Input: part model. Units: mm. Frame: model coordinates. Coordinates: 2 decimals unless noted, no trailing zeros. Write each loop counter-clockwise with the first axis right and the second up, starting at its lowest first coordinate (ties: lowest second). Pieces come first, ordered by that corner, then holes. Notation, with made-up numbers: M 52,83 L 107,83 A19 cw 107,95 Z; hole C 30,51 d6. An arc over 180 degrees is marked long. Use one line per item in the form item = value.
from build123d import *

# Parameters (mm, degrees)
SKETCH_1_W             = 270
SKETCH_1_H             = 107
SM_BASE_FLANGE_1_DEPTH = 5
SKETCH_6_R             = 3
CUT_EXTRUDE_1_DEPTH    = 10
SKETCH_7_R             = 1.5
CUT_EXTRUDE_2_DEPTH    = 10
FILLET_1_R             = 1
SKETCH_8_R             = 1.5
CUT_EXTRUDE_3_DEPTH    = 10


# Sheet-metal steps are written as plain solids
with BuildPart() as part:
    # Sketch 1 → 基体-法兰1 (new body)
    with BuildSketch(Plane.XY):
        Rectangle(SKETCH_1_W, SKETCH_1_H)
    extrude(amount=-SM_BASE_FLANGE_1_DEPTH)

    # 草图6 → 切除-拉伸1 (cut)
    with BuildSketch(Plane.XY):
        with Locations((-129, 35.5)):
            Circle(SKETCH_6_R)
        with Locations((-129, -35.5)):
            Circle(SKETCH_6_R)
        with Locations((-85, 35.5)):
            Circle(SKETCH_6_R)
        with Locations((-85, -35.5)):
            Circle(SKETCH_6_R)
    cut_extrude_1 = extrude(amount=-CUT_EXTRUDE_1_DEPTH, mode=Mode.SUBTRACT)

    # 镜向1: 切除-拉伸1 across plane
    add(cut_extrude_1.mirror(Plane(origin=(0, 0, 0), x_dir=(0, 0, 1), z_dir=(1, 0, 0))), mode=Mode.SUBTRACT)

    # 草图7 → 切除-拉伸2 (cut)
    with BuildSketch(Plane.XY):
        with Locations((0, 48.5)):
            Circle(SKETCH_7_R)
    cut_extrude_2 = extrude(amount=-CUT_EXTRUDE_2_DEPTH, mode=Mode.SUBTRACT)

    # 镜向2: 切除-拉伸2 across plane
    add(cut_extrude_2.mirror(Plane.ZX), mode=Mode.SUBTRACT)

    # 圆角1
    fillet_1_edges = [part.edges().sort_by_distance(p)[0] for p in [
        (135, -53.5, -2.5),
        (-135, -53.5, -2.5),
        (-135, 53.5, -2.5),
        (135, 53.5, -2.5),
    ]]
    fillet(fillet_1_edges, radius=FILLET_1_R)

    # 草图8 → 切除-拉伸3 (cut)
    with BuildSketch(Plane(origin=(0, 0, -5), x_dir=(-1, 0, 0), z_dir=(0, 0, -1))):
        with Locations((-5, 41.75)):
            Circle(SKETCH_8_R)
        with Locations((5, 41.75)):
            Circle(SKETCH_8_R)
        with Locations((5, 34.75)):
            Circle(SKETCH_8_R)
        with Locations((-5, 34.75)):
            Circle(SKETCH_8_R)
    cut_extrude_3 = extrude(amount=-CUT_EXTRUDE_3_DEPTH, mode=Mode.SUBTRACT)

    # 镜向3: 切除-拉伸3 across plane
    add(cut_extrude_3.mirror(Plane.ZX), mode=Mode.SUBTRACT)


solid = part.part
(1) First-contact query: pin 1 Ø4 at (x, y) = (5, 34.75) entering from -Z. Flat tip, straight axial feed; report the tip coordinate or a pass-through.
Computed:
pin_1 = -5
(2) Section query A-A on x = -129. Return the cut outline in (y, z), plus the area to 3 significant figures.
Computed:
outline = M -53.5,-5 L -38.5,-5 L -38.5,0 L -53.5,0 Z; M -32.5,-5 L 32.5,-5 L 32.5,0 L -32.5,0 Z; M 38.5,-5 L 53.5,-5 L 53.5,0 L 38.5,0 Z
area = 475 mm^2
(3) Line query: probe 1 along Y at (x, z) = (-5, -3); probe 2 along Y at (x, z) = (0, -2.4); probe 3 along Y at (x, z) = (-129, -1.1). Output: solid intervals per line, ascending.
Computed:
probe_1 = -53.5 to -43.25, -40.25 to -36.25, -33.25 to 33.25, 36.25 to 40.25, 43.25 to 53.5
probe_2 = -53.5 to -50, -47 to 47, 50 to 53.5
probe_3 = -53.5 to -38.5, -32.5 to 32.5, 38.5 to 53.5
(4) Pull-direction query (X, two-part tool) for faces 1 (the flat face through (-2, 1, 0)), 2 (the cylindrical face through (88, 35.6, -2.5)), 3 (the flat face through (135, -1, -2)), 4 (the flat face through (-135, -1, -2)); classes: pulls with the +X half, pulls with the -X half, needs draft (parallel to the pull), parting line crosses it, or undercut.
Computed:
face_1 = needs draft
face_2 = undercut
face_3 = pulls with the +X half
face_4 = pulls with the -X half
